Part model, mm, in its own coordinate system. Face numbers are marked on the shaded views. Round coordinates to 2 decimals unless told otherwise and drop trailing zeros. Write each loop counter-clockwise with the first axis right and the second up, starting at its lowest first coordinate (ties: lowest second). Pieces come first, ordered by that corner, then holes. Notation, with made-up numbers: (38.25, 42.5) -> (92.25, 42.5) arc R23 ccw to (92.25, 52.5) -> close; hole circle Ø9 at (80, 31.25). An arc over 180 degrees is marked (long way). Return JSON: item names as keys, results as strings. Group by question number.
(1) Saw through at A-A (z = 0). List the corners of the cut face in (x, y), plus the area to 4 significant figures.
(2) Saw through at B-B (x = -45). List the corners of the cut face in (y, z).
(3) Drill centre lines: L1, parallel to X at y = 300.75, z = -55; L2, parallel to Y at x = 10, z = 60; L3, parallel to Z at x = 45, y = 300. Where is each one in solid material? Low to high. Write a range as from..to.
(4) Saw through at D-D (y = 90). List the corners of the cut face in (x, z), plus the area to 3 significant figures.
(5) Saw through at C-C (x = 0). List the corners of the cut face in (y, z), plus the area to 4 significant figures.
(6) Drop flat-ended pins along their axis: pin 1 Ø10 at (x, z) = (45, 55) entering from -Y; pin 2 Ø1 at (y, z) = (42, 5) entering from -X; pin 3 Ø1 at (x, z) = (119, -38.5) entering from +Y. Give the stop position or say it passes through.
(7) Mould opens along Y. For the marked faces 1, 2 and 3 say: +Y half, -Y half, draft (parallel to the pull), parting line (faces both ways), or undercut.
from build123d import *

# Parameters (mm, degrees)
BOSS_EXTRUDE1_DEPTH = 25
SKETCH2_R           = 55
BOSS_EXTRUDE2_DEPTH = 265
SKETCH3_R           = 100
BOSS_EXTRUDE3_DEPTH = 15
SKETCH4_R           = 4.25
CUT_EXTRUDE1_DEPTH  = 15


with BuildPart() as part:
    # Sketch1 → Boss-Extrude1 (new body)
    with BuildSketch(Plane(origin=(0, 0, 0), x_dir=(1, 0, 0), z_dir=(0, 1, 0))):
        Polygon((-150, 130), (-130, 150), (130, 150), (150, 130), (150, -130), (130, -150), (-130, -150), (-150, -130), align=None)
    extrude(amount=BOSS_EXTRUDE1_DEPTH)

    # Sketch2 → Boss-Extrude2 (add)
    with BuildSketch(Plane(origin=(0, 25, 0), x_dir=(1, 0, 0), z_dir=(0, 1, 0))):
        Circle(SKETCH2_R)
    extrude(amount=BOSS_EXTRUDE2_DEPTH)

    # Sketch3 → Boss-Extrude3 (add)
    with BuildSketch(Plane(origin=(0, 290, 0), x_dir=(1, 0, 0), z_dir=(0, 1, 0))):
        Circle(SKETCH3_R)
    extrude(amount=BOSS_EXTRUDE3_DEPTH)

    # Sketch4 → Cut-Extrude1 (cut)
    with BuildSketch(Plane(origin=(0, 305, 0), x_dir=(1, 0, 0), z_dir=(0, 1, 0))):
        with Locations((-45, 55)):
            Circle(SKETCH4_R)
        with Locations((45, 55)):
            Circle(SKETCH4_R)
        with Locations((45, -55)):
            Circle(SKETCH4_R)
        with Locations((-45, -55)):
            Circle(SKETCH4_R)
    extrude(amount=-CUT_EXTRUDE1_DEPTH, mode=Mode.SUBTRACT)


solid = part.part
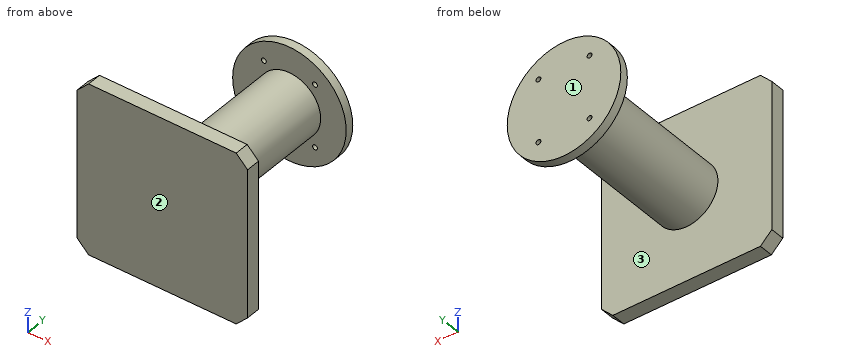
Computed values:
{
 "1": {"outline": "(-150, 0) -> (150, 0) -> (150, 25) -> (55, 25) -> (55, 290) -> (100, 290) -> (100, 305) -> (-100, 305) -> (-100, 290) -> (-55, 290) -> (-55, 25) -> (-150, 25) -> close", "area": "39,650 mm2"},
 "2": {"outline": "(0, -150) -> (25, -150) -> (25, -31.62) -> (290, -31.62) -> (290, -50.75) -> (305, -50.75) -> (305, 50.75) -> (290, 50.75) -> (290, 31.62) -> (25, 31.62) -> (25, 150) -> (0, 150) -> close; (290, -89.3) -> (305, -89.3) -> (305, -59.25) -> (290, -59.25) -> close; (290, 59.25) -> (305, 59.25) -> (305, 89.3) -> (290, 89.3) -> close"},
 "3": {"L1": "-83.52..-49.25, -40.75..40.75, 49.25..83.52", "L2": "0..25, 290..305", "L3": "-89.3..-59.25, -50.75..50.75, 59.25..89.3"},
 "4": {"outline": "circle Ø110 at (0, 0)", "area": "9,500 mm2"},
 "5": {"outline": "(0, -150) -> (25, -150) -> (25, -55) -> (290, -55) -> (290, -100) -> (305, -100) -> (305, 100) -> (290, 100) -> (290, 55) -> (25, 55) -> (25, 150) -> (0, 150) -> close", "area": "39,650 mm2"},
 "6": {"pin 1": "y = 0", "pin 2": "x = -54.82", "pin 3": "y = 25"},
 "7": {"face 1": "+Y half", "face 2": "-Y half", "face 3": "undercut"}
}
